```python
from build123d import *

# Parameters (mm, degrees)
BOSS_EXTRU_1_DEPTH       = 4
ENL_V_MAT_EXTRU_3_DEPTH  = 10
ESQUISSE3_R              = 2
ESQUISSE3_W              = 40
ESQUISSE3_H              = 20
ENL_V_MAT_EXTRU_4_DEPTH  = 242.33172191
ESQUISSE4_W              = 4
ESQUISSE4_H              = 200
ENL_V_MAT_EXTRU_5_DEPTH  = 242.33172191
ESQUISSE5_R              = 2.1
ENL_V_MAT_EXTRU_6_DEPTH  = 242.33172191
ESQUISSE8_W              = 5.4
ESQUISSE8_H              = 30.4
ENL_V_MAT_EXTRU_8_DEPTH  = 242.33172191
ESQUISSE10_W             = 4.4
ESQUISSE10_H             = 10.4
ENL_V_MAT_EXTRU_9_DEPTH  = 5
ESQUISSE12_R             = 2.1
BOSS_EXTRU_2_DEPTH       = 4
ESQUISSE14_W             = 14.6
ESQUISSE14_H             = 4
BOSS_EXTRU_3_DEPTH       = 4
ENL_V_MAT_EXTRU_11_DEPTH = 242.33172191
ENL_V_MAT_EXTRU_12_DEPTH = 242.33172191
ENL_V_MAT_EXTRU_13_DEPTH = 242.33172191
ENL_V_MAT_EXTRU_14_DEPTH = 242.33172191
ESQUISSE19_R             = 2.1
ENL_V_MAT_EXTRU_15_DEPTH = 242.33172191
ENL_V_MAT_EXTRU_16_DEPTH = 242.33172191


with BuildPart() as part:
    # Esquisse1 → Boss.-Extru.1 (new body)
    with BuildSketch(Plane.XY):
        Polygon((0, 0), (-135, 0), (-135, 200), (111, 200), (111, -80), (35, -80), align=None)
    extrude(amount=BOSS_EXTRU_1_DEPTH)

    # Esquisse2 → Enl_v. mat.-Extru.3 (cut)
    with BuildSketch(Plane(origin=(-100, 38, 4), x_dir=(-1, 0, 0), z_dir=(0, 0, -1))):
        with BuildLine():
            ThreePointArc((-75.787868531, -6.082649542), (-15.633697972, -12.332787722), (42.333333333, 4.912841999))
            ThreePointArc((42.333333333, 4.912841999), (44.422166387, 11.668341719), (37.666666667, 13.757174773))
            ThreePointArc((37.666666667, 13.757174773), (-16.560556167, -2.375833675), (-72.833812496, 3.471069783))
            ThreePointArc((-72.833812496, 3.471069783), (-79.087700176, 0.171238138), (-75.787868531, -6.082649542))
        make_face()
    extrude(amount=ENL_V_MAT_EXTRU_3_DEPTH, mode=Mode.SUBTRACT)

    # Esquisse3 → Enl_v. mat.-Extru.4 (cut, through all)
    with BuildSketch(Plane.XY.offset(4)):
        with Locations((-103.9, 185.1)):
            Circle(ESQUISSE3_R)
        with Locations((-103.9, 174.9)):
            Circle(ESQUISSE3_R)
        with Locations((-56.1, 185.1)):
            Circle(ESQUISSE3_R)
        with Locations((-56.1, 174.9)):
            Circle(ESQUISSE3_R)
        with Locations((-80, 180)):
            Rectangle(ESQUISSE3_W, ESQUISSE3_H)
    extrude(amount=-ENL_V_MAT_EXTRU_4_DEPTH, mode=Mode.SUBTRACT)

    # Esquisse4 → Enl_v. mat.-Extru.5 (cut, through all)
    with BuildSketch(Plane(origin=(0, 0, 0), x_dir=(-1, 0, 0), z_dir=(0, 0, -1))):
        with Locations((-109, 40)):
            Rectangle(ESQUISSE4_W, ESQUISSE4_H)
    extrude(amount=-ENL_V_MAT_EXTRU_5_DEPTH, mode=Mode.SUBTRACT)

    # Esquisse5 → Enl_v. mat.-Extru.6 (cut, through all)
    with BuildSketch(Plane(origin=(0, 0, 0), x_dir=(-1, 0, 0), z_dir=(0, 0, -1))):
        with Locations((-2.5, 180)):
            Circle(ESQUISSE5_R)
        with Locations((-2.5, 110)):
            Circle(ESQUISSE5_R)
        with Locations((-24.132044328, 83.658479689)):
            Circle(ESQUISSE5_R)
        with Locations((-87.332280645, 53.563129062)):
            Circle(ESQUISSE5_R)
    extrude(amount=-ENL_V_MAT_EXTRU_6_DEPTH, mode=Mode.SUBTRACT)

    # Esquisse8 → Enl_v. mat.-Extru.8 (cut, through all)
    with BuildSketch(Plane(origin=(0, 0, 0), x_dir=(-1, 0, 0), z_dir=(0, 0, -1))):
        Polygon((-40.847861933, 72.708071397), (-43.169503267, 77.583518198), (-70.616463039, 64.513537354), (-68.294821705, 59.638090553), align=None)
        with Locations((-2.5, 145)):
            Rectangle(ESQUISSE8_W, ESQUISSE8_H)
    extrude(amount=-ENL_V_MAT_EXTRU_8_DEPTH, mode=Mode.SUBTRACT)

    # Esquisse10 → Enl_v. mat.-Extru.9 (cut)
    with BuildSketch(Plane.ZY.offset(135)):
        with Locations((2, 95)):
            Rectangle(ESQUISSE10_W, ESQUISSE10_H)
        with Locations((2, 75.192593016)):
            Rectangle(ESQUISSE10_W, ESQUISSE10_H)
    extrude(amount=-ENL_V_MAT_EXTRU_9_DEPTH, mode=Mode.SUBTRACT)

    # Esquisse12 → Boss.-Extru.2 (add)
    with BuildSketch(Plane.XY.offset(4)):
        with BuildLine():
            Line((67.5, -80), (67.5, -82.5))
            ThreePointArc((67.5, -82.5), (72.5, -87.5), (77.5, -82.5))
            Line((77.5, -82.5), (77.5, -80))
            Line((77.5, -80), (67.5, -80))
        make_face()
        with Locations((72.5, -82.5)):
            Circle(ESQUISSE12_R, mode=Mode.SUBTRACT)
    extrude(amount=-BOSS_EXTRU_2_DEPTH)

    # Esquisse14 → Boss.-Extru.3 (add)
    with BuildSketch(Plane(origin=(0, 0, 0), x_dir=(-1, 0, 0), z_dir=(0, 0, -1))):
        with Locations((-42.5, -82)):
            Rectangle(ESQUISSE14_W, ESQUISSE14_H)
        with Locations((-102.5, -82)):
            Rectangle(ESQUISSE14_W, ESQUISSE14_H)
    extrude(amount=-BOSS_EXTRU_3_DEPTH)

    # Esquisse15 → Enl_v. mat.-Extru.11 (cut, through all)
    with BuildSketch(Plane(origin=(0, 0, 0), x_dir=(-1, 0, 0), z_dir=(0, 0, -1))):
        Polygon((-18.341719551, -41.923930403), (-16.658280449, -38.076069597), (-22.888150326, -35.350501525), (-22.327003958, -34.067881257), (-25.25870743, -32.785260988), (-25.819853798, -34.067881257), (-32.232955142, -31.262149418), (-33.916394245, -35.110010225), (-27.5032929, -37.915742063), (-28.064439268, -39.198362332), (-25.132735796, -40.480982601), (-24.571589429, -39.198362332), align=None)
    extrude(amount=-ENL_V_MAT_EXTRU_11_DEPTH, mode=Mode.SUBTRACT)

    # Esquisse16 → Enl_v. mat.-Extru.12 (cut, through all)
    with BuildSketch(Plane(origin=(0, 0, 0), x_dir=(-1, 0, 0), z_dir=(0, 0, -1))):
        Polygon((-111, 167.9), (-111, 172.1), (-104.2, 172.1), (-104.2, 173.5), (-101, 173.5), (-101, 172.1), (-94, 172.1), (-94, 167.9), (-101, 167.9), (-101, 166.5), (-104.2, 166.5), (-104.2, 167.9), align=None)
    extrude(amount=-ENL_V_MAT_EXTRU_12_DEPTH, mode=Mode.SUBTRACT)

    # Esquisse17 → Enl_v. mat.-Extru.13 (cut, through all)
    with BuildSketch(Plane(origin=(0, 0, 0), x_dir=(-1, 0, 0), z_dir=(0, 0, -1))):
        Polygon((69.6, 0), (65.4, 0), (65.4, 5.8), (64, 5.8), (64, 9), (65.4, 9), (65.4, 17), (69.6, 17), (69.6, 9), (71, 9), (71, 5.8), (69.6, 5.8), align=None)
    extrude(amount=-ENL_V_MAT_EXTRU_13_DEPTH, mode=Mode.SUBTRACT)

    # Esquisse18 → Enl_v. mat.-Extru.14 (cut, through all)
    with BuildSketch(Plane(origin=(0, 0, 0), x_dir=(-1, 0, 0), z_dir=(0, 0, -1))):
        Polygon((117.9, 200), (122.1, 200), (122.1, 193.2), (123.5, 193.2), (123.5, 190), (122.1, 190), (122.1, 183), (117.9, 183), (117.9, 190), (116.5, 190), (116.5, 193.2), (117.9, 193.2), align=None)
    extrude(amount=-ENL_V_MAT_EXTRU_14_DEPTH, mode=Mode.SUBTRACT)

    # Esquisse19 → Enl_v. mat.-Extru.15 (cut, through all)
    with BuildSketch(Plane.XY.offset(4)):
        with Locations((37.5, -23.25)):
            Circle(ESQUISSE19_R)
        with Locations((37.5, 43.25)):
            Circle(ESQUISSE19_R)
    extrude(amount=-ENL_V_MAT_EXTRU_15_DEPTH, mode=Mode.SUBTRACT)

    # Esquisse20 → Enl_v. mat.-Extru.16 (cut, through all)
    with BuildSketch(Plane(origin=(0, 0, 0), x_dir=(-1, 0, 0), z_dir=(0, 0, -1))):
        Polygon((130, 73.092593016), (130, 77.292593016), (124, 77.292593016), (124, 78.692593016), (120.8, 78.692593016), (120.8, 77.292593016), (113.8, 77.292593016), (113.8, 73.092593016), (120.8, 73.092593016), (120.8, 71.692593016), (124, 71.692593016), (124, 73.092593016), align=None)
    extrude(amount=-ENL_V_MAT_EXTRU_16_DEPTH, mode=Mode.SUBTRACT)


solid = part.part
```
Can you work these out from the model? Positions are in its coordinate system, mm. A direction names the side the tool comes from. Give positions to 0.01 mm unless a question says otherwise; leave off trailing zeros. Order: outer loops, then holes, each group sorted by start corner. A loop starts at its lowest first (then second) coordinate and runs counter-clockwise, first axis right, second up. Notation, with made-up numbers: M -23.75,42.25 L 21.25,42.25 A5 cw 21.25,49.25 Z; hole C 55,20 d5. An arc over 180 degrees is marked long. Write item = value, one per line. Start each with the question number.
Q1. For faces 1 (the flat face through (8.446, -19.305, 1.972)), 2 (the cylindrical face through (-82.72, 35.56, 2.03)), which set-ups out of +Z, -Z, +X, -X, +Y, -Y let a thin tool reach every point of the face, with its end or its side?
Q2. We'd pull the mould along Y, two halves only. Please class faces 3 (the flat face through (17, 90, 0)), 4 (the flat face through (26.79, -61.23, 1.97)), 5 (the flat face through (54.763, 66.082, 1.972)): pulls with the +Y half, pulls with the -Y half, needs draft (parallel to the pull), parting line crosses it, or undercut.
Q3. Suppose I cut it at A-A (y = -12). Write out the boundary of the cut face in (x, z).
Q4. I need wall thicknesses on probe 1 along Y at (x, z) = (-66, 0.3); probe 2 along X at (y, z) = (174.9, 3.05); probe 3 along X at (y, z) = (180, 1.2). Which ranges of each line are inside material? Lowest first, please. Write a range as [from, to].
Q5. Will these pins go through, and if not, where does the flat tip stop? pin 1 Ø2 at (x, z) = (-116, 2.5) entering from -Y; pin 2 Ø1.2 at (y, z) = (169.5, 2.5) entering from +X; pin 3 Ø1 at (x, z) = (54, 2.5) entering from -Y.
Q6. Suppose I cut it at B-B (z = 1.6). Count the separate pieces of the cut face and the enclosed holes in it, plus the area to 3 significant figures.
Check result:
q1.face_1 = +Z, -Z, -X, -Y
q1.face_2 = +Z, -Z
q2.face_3 = needs draft
q2.face_4 = pulls with the -Y half
q2.face_5 = undercut
q3.outline = M 5.25,0 L 107,0 L 107,4 L 5.25,4 Z
q4.probe_1 = [17, 25.05], [35.06, 170], [190, 200]
q4.probe_2 = [-135, -105.9], [-101.9, -100], [-60, -58.1], [-54.1, 111]
q4.probe_3 = [-135, -100], [-60, 0.4], [4.6, 111]
q5.pin_1 = 0
q5.pin_2 = 94
q5.pin_3 = -80
q6.separate_pieces = 1
q6.enclosed_holes = 14
q6.area = 53,100 mm2
